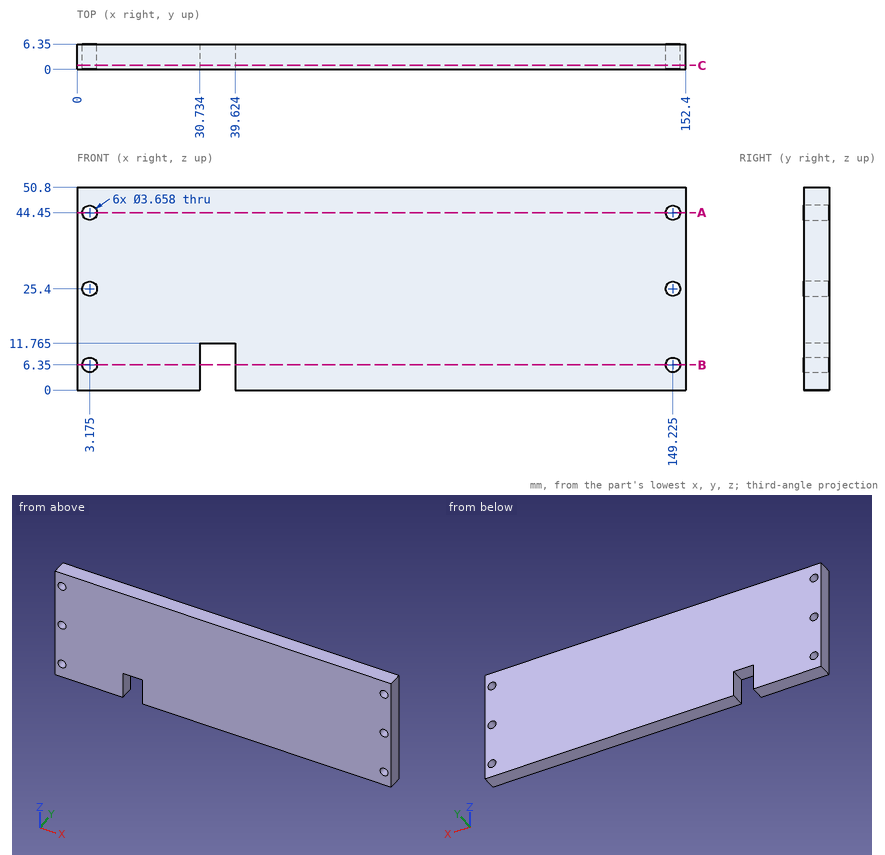
Print and shaded views of the part. All mm, measured from the part's lowest x, y and z. Give positions to 0.01 mm unless a question says otherwise; leave off trailing zeros. Loops run counter-clockwise (first coordinate to the right, second up) from the corner with the lowest first, then second, coordinate; pieces in that order, holes last. Notation, with made-up numbers: (-33, 52.25) -> (24, 52.25) arc R25 cw to (24, 73.25) -> close; hole circle Ø11 at (14, 56). An arc over 180 degrees is marked (long way). One line per question, with ' | ' between items. Start each with the question number.
1) Pin check, flat tip, straight feed: pin 1 (5 mm diameter, centred on x = 3.175, z = 44.45, fed in from -Y). Stop position of the tip, or through.
2) Cut at C-C (y = 1). Count the separate pieces of the cut face and the enclosed holes in it, plus the area to 3 significant figures.
3) Probe L1, parallel to X at y = 5.25, z = 44.45; L2, parallel to X at y = 5, z = 8 (1 decimal); L3, parallel to X at y = 1, z = 46 (1 decimal). List the from-to ranges inside material, lowest first.
4) Cut at B-B (z = 6.35). Give the cut face in (x, y).
5) Cut at A-A (z = 44.45). Give the cut face in (x, y).
Return value:
1) pin 1: y = 0
2) separate pieces: 1 | enclosed holes: 6 | area: 7,570 mm^2
3) L1: 0 to 1.35, 5 to 147.4, 151.05 to 152.4 | L2: 0 to 2.4, 4 to 30.7, 39.6 to 148.4, 150 to 152.4 | L3: 0 to 2.2, 4.1 to 148.3, 150.2 to 152.4
4) outline: (0, 0) -> (1.35, 0) -> (1.35, 6.35) -> (0, 6.35) -> close; (5, 0) -> (30.73, 0) -> (30.73, 6.35) -> (5, 6.35) -> close; (39.62, 0) -> (147.4, 0) -> (147.4, 6.35) -> (39.62, 6.35) -> close; (151.05, 0) -> (152.4, 0) -> (152.4, 6.35) -> (151.05, 6.35) -> close
5) outline: (0, 0) -> (1.35, 0) -> (1.35, 6.35) -> (0, 6.35) -> close; (5, 0) -> (147.4, 0) -> (147.4, 6.35) -> (5, 6.35) -> close; (151.05, 0) -> (152.4, 0) -> (152.4, 6.35) -> (151.05, 6.35) -> close
